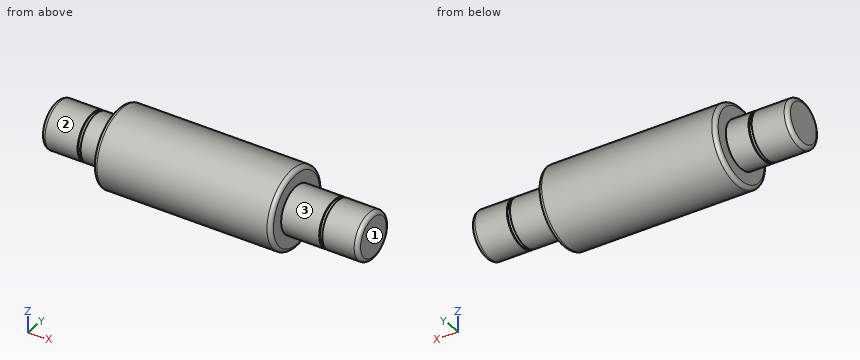
```python
from build123d import *

# Parameters (mm, degrees)
SKETCH2_R           = 5
SKETCH2_R_2         = 3
CUT_EXTRUDE2_DEPTH  = 1.9
FILLET1_R           = 0.5
BOSS_EXTRUDE2_START = 0.1
SKETCH4_R           = 3
SKETCH4_R_2         = 2.85
BOSS_EXTRUDE2_DEPTH = 0.1
SKETCH6_R           = 3
SKETCH6_R_2         = 2.85
BOSS_EXTRUDE3_DEPTH = 0.02
BOSS_EXTRUDE4_START = 0.08
SKETCH7_R           = 3
SKETCH7_R_2         = 2.85
BOSS_EXTRUDE4_DEPTH = 0.08


with BuildPart() as part:
    # Sketch1 → Revolve1 (revolve)
    with BuildSketch(Plane.XY, mode=Mode.PRIVATE) as revolve1_sk:
        Polygon((-12.4, 5), (12.4, 5), (12.4, 3), (15.32, 3), (15.32, 2.85), (15.82, 2.85), (15.82, 3), (20.4, 3), (20.4, 0), (-20.4, 0), (-20.4, 3), (-15.82, 3), (-15.82, 2.85), (-15.32, 2.85), (-15.32, 3), (-12.4, 3), align=None)
    revolve(revolve1_sk.sketch.rotate(Axis((-20.4, 0, 0), (1, 0, 0)), 180), axis=Axis((-20.4, 0, 0), (1, 0, 0)))

    # Sketch2 → Cut-Extrude2 (cut)
    with BuildSketch(Plane(origin=(12.4, 0, 0), x_dir=(0, 0, -1), z_dir=(1, 0, 0))):
        with Locations(Location((0, 0, 0), (0, 0, 270))):
            Circle(SKETCH2_R)
        with Locations(Location((0, 0, 0), (0, 0, 270))):
            Circle(SKETCH2_R_2, mode=Mode.SUBTRACT)
    extrude(amount=-CUT_EXTRUDE2_DEPTH, mode=Mode.SUBTRACT)

    # Fillet1
    fillet1_edges = [part.edges().sort_by_distance(p)[0] for p in [
        (20.4, 3, 0),
        (-20.4, 3, 0),
        (-12.4, 5, 0),
        (10.5, 5, 0),
    ]]
    fillet(fillet1_edges, radius=FILLET1_R)

    # Sketch4 → Boss-Extrude2 (add)
    with BuildSketch(Plane(origin=(-15.82, 0, 0), x_dir=(0, 0, -1), z_dir=(1, 0, 0)).offset(BOSS_EXTRUDE2_START)):
        with Locations(Location((0, 0, 0), (0, 0, 270))):
            Circle(SKETCH4_R)
        with Locations(Location((0, 0, 0), (0, 0, 270))):
            Circle(SKETCH4_R_2, mode=Mode.SUBTRACT)
    extrude(amount=-BOSS_EXTRUDE2_DEPTH)

    # Sketch6 → Boss-Extrude3 (add)
    with BuildSketch(Plane.ZY.offset(-15.82)):
        with Locations(Location((0, 0, 0), (0, 0, 270))):
            Circle(SKETCH6_R)
        with Locations(Location((0, 0, 0), (0, 0, 270))):
            Circle(SKETCH6_R_2, mode=Mode.SUBTRACT)
    extrude(amount=BOSS_EXTRUDE3_DEPTH)

    # Sketch7 → Boss-Extrude4 (add)
    with BuildSketch(Plane(origin=(15.32, 0, 0), x_dir=(0, 0, -1), z_dir=(1, 0, 0)).offset(BOSS_EXTRUDE4_START)):
        with Locations(Location((0, 0, 0), (0, 0, 270))):
            Circle(SKETCH7_R)
        with Locations(Location((0, 0, 0), (0, 0, 270))):
            Circle(SKETCH7_R_2, mode=Mode.SUBTRACT)
    extrude(amount=-BOSS_EXTRUDE4_DEPTH)


solid = part.part
```
Geometry check sheet. Reference: the model listing, model coordinates, mm. Face numbers are marked on the shaded views. A direction names the side the tool comes from. Give positions to 0.01 mm unless a question says otherwise; leave off trailing zeros. Write each loop counter-clockwise with the first axis right and the second up, starting at its lowest first coordinate (ties: lowest second). Pieces come first, ordered by that corner, then holes. Notation, with made-up numbers: (32, 53.5) -> (88, 53.5) arc R23 cw to (88, 83.5) -> close; hole circle Ø11 at (16.25, -27.75). An arc over 180 degrees is marked (long way). Use one line per item in the form item = value.
Item 1: Scan lines: line 1 (Y direction, x = 7.5, z = -0.25); line 2 (X direction, y = 2.5, z = -3.75); line 3 (Y direction, x = 3, z = 4). Record each from-to range of solid material in increasing order.
Results list:
line_1 = -4.99 to 4.99
line_2 = -12.4 to 10.5
line_3 = -3 to 3
Item 2: Depth check by flat-ended pin: pin 1 Ø3 at (y, z) = (-2.5, -3.5) entering from -X; pin 2 Ø2 at (y, z) = (-3.5, 3.5) entering from -X; pin 3 Ø3 at (x, z) = (-10.5, -3) entering from +Y. Enter the tip coordinate at first touch or a pass-through.
Results list:
pin_1 = -20.3
pin_2 = -12.4
pin_3 = 4.77
Item 3: Access from +Z, -Z, +X, -X, +Y, -Y to the whole of each face (thin tool, end or side, straight path). Record for the marked faces 1, 2 and 3.
Results list:
face_1 = +Z, -Z, +X, +Y, -Y
face_2 = -X
face_3 = +X
Item 4: Sectioned sample at A-A on x = -5. Enter the section's corners in (y, z).
Results list:
outline = circle Ø10 at (0, 0)
